from build123d import *

# Parameters (mm, degrees)
SKETCH1_W           = 430
SKETCH1_H           = 430
BOSS_EXTRUDE1_DEPTH = 0.45
SKETCH7_R           = 3.3
BOSS_EXTRUDE2_DEPTH = 5
SKETCH8_R           = 1.75
CUT_EXTRUDE1_DEPTH  = 4
SKETCH6_R           = 3.3
BOSS_EXTRUDE3_DEPTH = 5
SKETCH10_R          = 1.75
CUT_EXTRUDE2_DEPTH  = 4


with BuildPart() as part:
    # Sketch1 → Boss-Extrude1 (new body)
    with BuildSketch(Plane(origin=(0, 0, 0), x_dir=(1, 0, 0), z_dir=(0, 1, 0))):
        Rectangle(SKETCH1_W, SKETCH1_H)
    extrude(amount=BOSS_EXTRUDE1_DEPTH)

    # Sketch7 → Boss-Extrude2 (add)
    with BuildSketch(Plane(origin=(0, 0.45, 0), x_dir=(1, 0, 0), z_dir=(0, 1, 0))):
        with Locations(Location((-116.362714529, 94.945868521, 0), (0, 0, 90))):
            Circle(SKETCH7_R)
        with Locations(Location((-55.363204635, 95.191638193, 0), (0, 0, 90))):
            Circle(SKETCH7_R)
        with Locations(Location((-54.980448566, 0.192396061, 0), (0, 0, 90))):
            Circle(SKETCH7_R)
        with Locations(Location((-115.97995846, -0.053373612, 0), (0, 0, 90))):
            Circle(SKETCH7_R)
    extrude(amount=BOSS_EXTRUDE2_DEPTH)

    # Sketch8 → Cut-Extrude1 (cut)
    with BuildSketch(Plane(origin=(0, 5.45, 0), x_dir=(1, 0, 0), z_dir=(0, 1, 0))):
        with Locations(Location((-54.980448566, 0.192396061, 0), (0, 0, 270))):
            Circle(SKETCH8_R)
        with Locations(Location((-55.363204635, 95.191638193, 0), (0, 0, 270))):
            Circle(SKETCH8_R)
        with Locations(Location((-116.362714529, 94.945868521, 0), (0, 0, 270))):
            Circle(SKETCH8_R)
        with Locations(Location((-115.97995846, -0.053373612, 0), (0, 0, 270))):
            Circle(SKETCH8_R)
    extrude(amount=-CUT_EXTRUDE1_DEPTH, mode=Mode.SUBTRACT)

    # Sketch6 → Boss-Extrude3 (add)
    with BuildSketch(Plane(origin=(0, 0.45, 0), x_dir=(1, 0, 0), z_dir=(0, 1, 0))):
        with Locations(Location((119.793345796, 46.373061352, 0), (0, 0, 90))):
            Circle(SKETCH6_R)
        with Locations(Location((69.793345796, 46.373061352, 0), (0, 0, 90))):
            Circle(SKETCH6_R)
        with Locations(Location((119.793345796, -103.626938648, 0), (0, 0, 90))):
            Circle(SKETCH6_R)
        with Locations(Location((69.793345796, -103.626938648, 0), (0, 0, 90))):
            Circle(SKETCH6_R)
    extrude(amount=BOSS_EXTRUDE3_DEPTH)

    # Sketch10 → Cut-Extrude2 (cut)
    with BuildSketch(Plane(origin=(0, 5.45, 0), x_dir=(1, 0, 0), z_dir=(0, 1, 0))):
        with Locations(Location((69.793345796, 46.373061352, 0), (0, 0, 270))):
            Circle(SKETCH10_R)
        with Locations(Location((119.793345796, 46.373061352, 0), (0, 0, 270))):
            Circle(SKETCH10_R)
        with Locations(Location((119.793345796, -103.626938648, 0), (0, 0, 270))):
            Circle(SKETCH10_R)
        with Locations(Location((69.793345796, -103.626938648, 0), (0, 0, 270))):
            Circle(SKETCH10_R)
    extrude(amount=-CUT_EXTRUDE2_DEPTH, mode=Mode.SUBTRACT)


solid = part.part
CAD build for the part. Positions are in the model's coordinates, mm. Give positions to 0.01 mm unless a question says otherwise; leave off trailing zeros. Order: outer loops, then holes, each group sorted by start corner. A loop starts at its lowest first (then second) coordinate and runs counter-clockwise, first axis right, second up. Notation, with made-up numbers: (25.5, 87.5) -> (29.5, 87.5) arc R30 cw to (29.5, 117.5) -> close; hole circle Ø6 at (-30.75, 67). An arc over 180 degrees is marked (long way). Return JSON: item names as keys, results as strings.
Q1. Drill centre lines: line 1 (X direction, y = 2.7, z = -94); line 2 (Y direction, x = -38.5, z = -13). Where is each one in solid material? Low to high.
Working result:
{"line 1": "-119.52 to -117.84, -114.89 to -113.2, -58.44 to -56.64, -54.08 to -52.29", "line 2": "0 to 0.45"}
Q2. Flat gauge pins, fed straight in: pin 1 (2 mm diameter, centred on x = -54.98, z = -0.19, fed in from +Y); pin 2 (8 mm diameter, centred on x = -6.5, z = 158.5, fed in from +Y); pin 3 (2 mm diameter, centred on x = 68, y = 4.5, fed in from +Z). Where does each tip first touch, or does it go through?
Working result:
{"pin 1": "y = 1.45", "pin 2": "y = 0.45", "pin 3": "z = 106.83"}
Q3. Saw through at B-B (x = -171). Write the cut outline in (y, z).
Working result:
{"outline": "(0, -215) -> (0.45, -215) -> (0.45, 215) -> (0, 215) -> close"}
Q4. Saw through at A-A (y = 4.2). Count the separate pieces of the cut face and the enclosed holes in it, then the cut area to 3 significant figures.
Working result:
{"separate pieces": "8", "enclosed holes": "8", "area": "197 mm²"}
Q5. Saw through at C-C (z = 155.5). Write the cut outline in (x, y).
Working result:
{"outline": "(-215, 0) -> (215, 0) -> (215, 0.45) -> (-215, 0.45) -> close"}
